The listing builds one solid part. Answer for the finished solid, in the listing's coordinates (mm). A direction names the side the tool comes from. Give positions to 0.01 mm unless a question says otherwise; leave off trailing zeros. Write each loop counter-clockwise with the first axis right and the second up, starting at its lowest first coordinate (ties: lowest second). Pieces come first, ordered by that corner, then holes. Notation, with made-up numbers: (36.5, 55.5) - (66.5, 55.5) arc R17 cw to (66.5, 77.5) - close; hole circle Ø9 at (63.5, 1.25). An arc over 180 degrees is marked (long way). Return JSON: item names as keys, results as strings.
from build123d import *

# Parameters (mm, degrees)
SKETCH1_W           = 35
SKETCH1_H           = 4
SKETCH1_H_2         = 16
BOSS_EXTRUDE1_DEPTH = 3
SKETCH1_3_W         = 35
SKETCH1_3_H         = 4
BOSS_EXTRUDE2_DEPTH = 21


with BuildPart() as part:
    # Sketch1 → Boss-Extrude1 (new body)
    with BuildSketch(Plane(origin=(0, 0, 0), x_dir=(1, 0, 0), z_dir=(0, 1, 0))):
        with Locations((0, 8)):
            Rectangle(SKETCH1_W, SKETCH1_H)
        with Locations((0, -2)):
            Rectangle(SKETCH1_W, SKETCH1_H_2)
    extrude(amount=BOSS_EXTRUDE1_DEPTH)

    # Sketch1_3 → Boss-Extrude2 (add)
    with BuildSketch(Plane(origin=(0, 0, 0), x_dir=(1, 0, 0), z_dir=(0, 1, 0))):
        with Locations((0, 8)):
            Rectangle(SKETCH1_3_W, SKETCH1_3_H)
    extrude(amount=BOSS_EXTRUDE2_DEPTH)


solid = part.part
Item 1: For faces 1 (the face through (0, 3, 2)), 2 (the face through (0, 0, 0)), determine the directions among +Z, -Z, +X, -X, +Y, -Y from which every point of the face is accessible in a straight line to the end or side of a thin tool.
Answer below:
{"face 1": "+Z, +X, -X, +Y", "face 2": "+Z, -Z, +X, -X, -Y"}
Item 2: A cutting plane is placed at B-B on z = -1.25. Determine the outline of the cut face in (x, y), then the cut area to 3 significant figures.
Answer below:
{"outline": "(-17.5, 0) - (17.5, 0) - (17.5, 3) - (-17.5, 3) - close", "area": "105 mm²"}
Item 3: Flat-ended cylindrical pins translate along their axes: P1, Ø5, axis at x = -4, z = -1, coming from the +Y side; P2, Ø3, axis at x = 8, y = 15.5, coming from the +Z side. Find the tip coordinate at first contact, or state that the pin passes through.
Answer below:
{"P1": "stops at y = 3", "P2": "stops at z = -6"}
Item 4: Consider L1, parallel to Y at x = -1.5, z = 2.5; L2, parallel to Z at x = -10, y = 19. Determine where each line is inside the solid, lowest interval first.
Answer below:
{"L1": "y = 0 to 3", "L2": "z = -10 to -6"}
Item 5: A cutting plane is placed at A-A on x = -6. Determine the outline of the cut face in (y, z).
Answer below:
{"outline": "(0, -10) - (21, -10) - (21, -6) - (3, -6) - (3, 10) - (0, 10) - close"}
Item 6: A cutting plane is placed at C-C on y = 11.75. Determine the outline of the cut face in (x, z).
Answer below:
{"outline": "(-17.5, -10) - (17.5, -10) - (17.5, -6) - (-17.5, -6) - close"}
